Work out the finished part from the listing and answer in its coordinate system (mm). A direction names the side the tool comes from. Round coordinates to 2 decimals unless told otherwise and drop trailing zeros. Order: outer loops, then holes, each group sorted by start corner. A loop starts at its lowest first (then second) coordinate and runs counter-clockwise, first axis right, second up. Notation, with made-up numbers: (30, 70) -> (39, 70) arc R25 cw to (39, 95) -> close; hole circle Ø9 at (-15.75, 46.5). An arc over 180 degrees is marked (long way). Use one line per item in the form item = value.
```python
from build123d import *

# Parameters (mm, degrees)
SKETCH028_W  = 13
SKETCH028_H  = 45
PAD026_DEPTH = 8.5
SKETCH030_W  = 15
SKETCH030_H  = 45
PAD028_DEPTH = 70.5


with BuildPart() as body029:
    # Sketch028 → Pad026 (new body)
    with BuildSketch(Plane.XY):
        with Locations((-28.5, -16.5)):
            Rectangle(SKETCH028_W, SKETCH028_H)
    extrude(amount=PAD026_DEPTH)


with BuildPart() as body029_1:
    # Body029 placement: moved
    add(body029.part.moved(Location((-1, -21.5, 2))))


with BuildPart() as cut030:
    # Sketch030 → Pad028 (new body)
    with BuildSketch(Plane.XY):
        with Locations((-27.5, -16.5)):
            Rectangle(SKETCH030_W, SKETCH030_H)
    extrude(amount=PAD028_DEPTH)


with BuildPart() as cut030_1:
    # Body031 placement: moved
    add(cut030.part.moved(Location((-3, -21.5, -58))))

    # Cut030: cut Body029
    add(body029_1.part, mode=Mode.SUBTRACT)


solid = cut030_1.part
```
Item 1: The part is cut by section C-C, the plane z = 3.5. Give the vertices of the cut face in (x, y), and give its area (3 significant figures).
Findings:
outline = (-38, -60.5) -> (-36, -60.5) -> (-36, -15.5) -> (-38, -15.5) -> close
area = 90.0 mm^2
Item 2: The part is cut by section A-A, the plane x = -32. Give the vertices of the cut face in (y, z), and give its area (3 significant figures).
Findings:
outline = (-60.5, -58) -> (-15.5, -58) -> (-15.5, 2) -> (-60.5, 2) -> close; (-60.5, 10.5) -> (-15.5, 10.5) -> (-15.5, 12.5) -> (-60.5, 12.5) -> close
area = 2,790 mm^2
Item 3: Determine the mould class of faces 3 (the flat face through (-31, -15.5, -23)), 4 (the flat face through (-31, -38, -58)), 5 (the flat face through (-36, -38, 6)), 6 (the flat face through (-30, -38, 10.5)) for opening direction Z: released by +Z, released by -Z, zero draft, split by the parting line, or undercut.
Findings:
face_3 = zero draft
face_4 = released by -Z
face_5 = undercut
face_6 = undercut
Item 4: For faces 1 (the flat face through (-31, -60.5, -23)), 2 (the flat face through (-30, -38, 2)), determine the directions among +Z, -Z, +X, -X, +Y, -Y from which every point of the face is accessible in a straight line to the end or side of a thin tool.
Findings:
face_1 = +Z, -Z, +X, -X, -Y
face_2 = +X, +Y, -Y
Item 5: Consider line 1 along Z through (x, y) = (-25.75, -33.5); line 2 along X through (y, z) = (-42, 4). Determine where each line is inside the solid, lowest interval first.
Findings:
line_1 = -58 to 2, 10.5 to 12.5
line_2 = -38 to -36
Item 6: A flat-ended cylindrical pin translates along its axis: P1, Ø2.5, axis at y = -48, z = 4, coming from the +X side. Find the tip coordinate at first contact, or state that the pin passes through.
Findings:
P1 = -36
Item 7: The part is cut by section B-B, the plane y = -42.5. Give the vertices of the cut face in (x, z), and give its area (3 significant figures).
Findings:
outline = (-38, -58) -> (-23, -58) -> (-23, 2) -> (-36, 2) -> (-36, 10.5) -> (-23, 10.5) -> (-23, 12.5) -> (-38, 12.5) -> close
area = 947 mm^2
